```python
from build123d import *

# Parameters (mm, degrees)
F1_DEPTH     = 25
F3_W         = 103.0636096465
F3_H         = 15
F3_W_2       = 5
F3_W_3       = 5.0301977637
F4_DEPTH     = 29.1
F5_W         = 32.1414392277
F5_H         = 15
F5_W_2       = 37.424231063
F6_DEPTH     = 5
F8_W         = 35.7737973711
F8_H         = 15
F9_DEPTH     = 25
F10_T1_DEPTH = 45.720844557
F11_R        = 1
F12_W        = 15.2368300635
F12_H        = 15
F13_DEPTH    = 30


# Not quite as in the source:
# - a fillet or chamfer that OpenCascade refuses, or shapes differently, is made with other operations: its cross-section is extruded or revolved along the edge and cut away or added


with BuildPart() as f1:
    # F0 (on Top) → F1 (new body)
    with BuildSketch(Plane.XY):
        Polygon((-57.4114776212, 45), (-65.7924397243, 0), (139.809737024, 0), (141.2981229206, 7.9916081853), (136.3826469731, 8.9070841327), align=None)
        Polygon((18.9005100522, 25.701403032), (130.0528008015, 5), (-12.1503930873, 5), (-21.1640298367, 5), (-27.6338049994, 5), (-59.7752442271, 5), (-53.8331571099, 36.9049193859), (-53.4114776212, 39.1690481052), (-48.4663143975, 38.2480430925), (11.8550538619, 27.0135741727), align=None, mode=Mode.SUBTRACT)
        Polygon((136.3826469731, 8.9070841327), (141.2981229206, 7.9916081853), (141.2981229206, 14.3588015401), (137.528741777, 15.0608246626), align=None)
        Polygon((-27.6338049994, 5), (-21.1640298367, 5), (-48.4663143975, 38.2480430925), (-53.4114776212, 39.1690481052), (-53.8331571099, 36.9049193859), align=None)
        Polygon((-12.1503930873, 5), (18.9005100522, 25.701403032), (11.8550538619, 27.0135741727), (-21.1640298367, 5), align=None)
    extrude(amount=F1_DEPTH)

    # F3 (on offset) → F4 (cut)
    with BuildSketch(Plane(origin=(6.1753463271, 33.1573608496, 0), x_dir=(-0.9830951895, 0.1830951895, 0), z_dir=(0.1830951895, 0.9830951895, 0))):
        with Locations((-70.4070020763, 12.5)):
            Rectangle(F3_W, F3_H)
        Polygon((49.6500332337, 20), (-1.7085909409, 20), (-1.7085909409, 5), (0, 5), (49.6500332337, 5), align=None)
        with Locations((-124.4388068995, 12.5)):
            Rectangle(F3_W_2, F3_H)
        with Locations((-16.375197253, 12.5)):
            Rectangle(F3_W_2, F3_H)
        Polygon((-1.7085909409, 20), (-6.7085909409, 20), (-6.7085909409, 0), (54.6500332337, 0), (54.6500332337, 5), (49.6500332337, 5), (0, 5), (-1.7085909409, 5), align=None)
        with Locations((52.1500332337, 12.5)):
            Rectangle(F3_W_2, F3_H)
        with Locations((57.1651321155, 12.5)):
            Rectangle(F3_W_3, F3_H)
    extrude(amount=-F4_DEPTH, mode=Mode.SUBTRACT)

    # F5 (on Front) → F6 (cut)
    with BuildSketch(Plane.XZ):
        with Locations((-43.7045246133, 12.5)):
            Rectangle(F5_W, F5_H)
        with Locations((6.5617224442, 12.5)):
            Rectangle(F5_W_2, F5_H)
    extrude(amount=-F6_DEPTH, mode=Mode.SUBTRACT)

    # F8 (on offset) → F9 (cut)
    with BuildSketch(Plane(origin=(-63.5868239483, 11.8426391504, 0), x_dir=(-0.1830951895, -0.9830951895, 0), z_dir=(-0.9830951895, 0.1830951895, 0))):
        with Locations((-10.8406194676, 12.5)):
            Rectangle(F8_W, F8_H)
    extrude(amount=-F9_DEPTH, mode=Mode.SUBTRACT)

    # F10: fillet of radius 5 on 1 edges, made by hand

    # F10_s2 → F10_t1 (cut)
    with BuildSketch(Plane.XY.offset(-10.3604222785)):
        with BuildLine():
            ThreePointArc((141.2981229206, 10.2146326287), (140.2448363813, 13.2843969289), (137.528741777, 15.0608246626))
            Line((137.528741777, 15.0608246626), (141.2981229206, 14.3588015401))
            Line((141.2981229206, 14.3588015401), (141.2981229206, 10.2146326287))
        make_face()
    extrude(amount=F10_T1_DEPTH, mode=Mode.SUBTRACT)

    # F11
    f11_edges = [f1.edges().sort_by_distance(p)[0] for p in [
        (137.528742, 15.060825, 12.5),
    ]]
    fillet(f11_edges, radius=F11_R)

    # F12 (on Right) → F13 (cut)
    with BuildSketch(Plane.YZ):
        with Locations((12.5338909792, 12.5)):
            Rectangle(F12_W, F12_H)
    extrude(amount=-F13_DEPTH, mode=Mode.SUBTRACT)


solid = f1.part
```
The listing builds one solid part. Answer for the finished solid, in the listing's coordinates (mm). A direction names the side the tool comes from. Give positions to 0.01 mm unless a question says otherwise; leave off trailing zeros. Order: outer loops, then holes, each group sorted by start corner. A loop starts at its lowest first (then second) coordinate and runs counter-clockwise, first axis right, second up. Notation, with made-up numbers: (-9.5, 30) -> (23.5, 30) arc R15 ccw to (23.5, 38) -> close; hole circle Ø2 at (16, -13.75). An arc over 180 degrees is marked (long way). Answer as CSV lines item,"result". Start each with the question number.
Q1. A cutting plane is placed at D-D (x = 93.5). Determine the outline of the cut face in (y, z).
Q2. A cutting plane is placed at B-B (x = 14.5). Determine the outline of the cut face in (y, z).
Q3. Determine the mould class of faces 1 (the flat face through (22, 4, 25)), 2 (the flat face through (-61.543, 22.815, 20.658)), 3 (the flat face through (-43, 5, 22)) for opening direction X: pulls with the +X half, pulls with the -X half, needs draft (parallel to the pull), parting line crosses it, or undercut.
Q4. Given pin 1 (2.5 mm diameter, centred on x = -37, z = 1.5, fed in from +Y); pin 2 (12 mm diameter, centred on x = -41, y = 23, fed in from -Z); pin 3 (8 mm diameter, centred on y = 21, z = 8.5, fed in from -X), each flat-ended and moving along its own axis, determine where each tip first touches the part or whether it passes through.
Q5. A cutting plane is placed at A-A (z = 16.5). Determine the outline of the cut face in (x, y), then the cut area to 3 significant figures.
Q6. Which of the six approach directions +Z, -Z, +X, -X, +Y, -Y give full straight-line access (tool end or side, diameter ignored) to faces 4 (the flat face through (-56.846, 20.729, 2.465)), 5 (the flat face through (130.06, 5.03, 12.4)), 6 (the flat face through (-52.947, 41.661, 12.395))?
Q7. Find the intervals of material crossed by L1, parallel to Z at x = -40, y = 38; L2, parallel to Y at x = 104, z = 21.5; L3, parallel to Y at x = -13, z = 21, in increasing order.
Q8. A cutting plane is placed at C-C (y = 22.5). Determine the outline of the cut face in (x, z), then the cut area to 3 significant figures.
Results found:
1,outline,"(0, 0) -> (5, 0) -> (5, 5) -> (0, 5) -> close; (0, 20) -> (5, 20) -> (5, 25) -> (0, 25) -> close; (11.81, 0) -> (16.89, 0) -> (16.89, 5) -> (11.81, 5) -> close; (11.81, 20) -> (16.89, 20) -> (16.89, 25) -> (11.81, 25) -> close"
2,outline,"(0, 0) -> (5, 0) -> (5, 5) -> (0, 5) -> close; (0, 20) -> (5, 20) -> (5, 25) -> (0, 25) -> close; (22.77, 0) -> (31.61, 0) -> (31.61, 25) -> (22.77, 25) -> close"
3,face 1,"needs draft"
3,face 2,"pulls with the -X half"
3,face 3,"undercut"
4,pin 1,"y = 5"
4,pin 2,"z = 20"
4,pin 3,"x = -62.24"
5,outline,"(-65.79, 0) -> (-59.78, 0) -> (-59.78, 3.97) -> (-64.88, 4.92) -> close; (-58.33, 40.08) -> (-53.41, 39.17) -> (-52.5, 44.08) -> (-57.41, 45) -> close; (-32.34, 10.73) -> (-30, 7.88) -> (-30, 10.29) -> close; (-27.63, 0) -> (-12.15, 0) -> (-12.15, 4.92) -> (-27.63, 4.92) -> close; (10.58, 20.15) -> (18.9, 25.7) -> (19.82, 30.62) -> (12.77, 31.93) -> close; (129.12, 0) -> (139.81, 0) -> (141.3, 7.99) -> (141.3, 10.21) arc R5 ccw to (138.79, 14.55) arc R1 ccw to (137.31, 13.87) -> (136.38, 8.91) -> (130.97, 9.92) -> close"
5,area,"309 mm2"
6,face 4,"+Z, -Z"
6,face 5,"+Y"
6,face 6,"+X, -Y"
7,L1,"20 to 25"
7,L2,"0 to 5, 9.85 to 14.94"
7,L3,"0 to 10.44, 31.64 to 36.73"
8,outline,"(-61.6, 0) -> (-56.52, 0) -> (-56.52, 5) -> (-61.6, 5) -> close; (-61.6, 20) -> (-56.52, 20) -> (-56.52, 25) -> (-61.6, 25) -> close; (-42, 20) -> (-35.53, 20) -> (-35.53, 25) -> (-42, 25) -> close; (5.08, 20) -> (11.01, 20) -> (11.01, 0) -> (14.1, 0) -> (14.1, 25) -> (5.08, 25) -> close; (36.09, 0) -> (63.4, 0) -> (63.4, 5) -> (36.09, 5) -> close; (36.09, 20) -> (63.4, 20) -> (63.4, 25) -> (36.09, 25) -> close"
8,area,"463 mm2"
